The model under review builds one solid part; all positions refer to its coordinate system, in mm. A direction names the side the tool comes from. Coordinates: 2 decimals unless noted, no trailing zeros. Loops run counter-clockwise (first coordinate to the right, second up) from the corner with the lowest first, then second, coordinate; pieces in that order, holes last. Notation, with made-up numbers: (22, -16) - (78, -16) arc R19 cw to (78, 3) - close; hole circle Ø3 at (34.5, 59). An arc over 180 degrees is marked (long way). Answer in a Markdown table with one row per item. Add a question column.
(1) For line 1 along X through (y, z) = (-0.5, 1.45); line 2 along Z through (x, y) = (-2, -1.5); line 3 along X through (y, z) = (3.75, 2.3), list the stretches that pass through material, from the lowest coordinate up.
(2) Machinability: for faces 4 (the flat face through (1.3, -0.1, 1.8)), 5 (the flat face through (-0.21, -5, 0.48)), which of the approach directions +Z, -Z, +X, -X, +Y, -Y give a long, thin tool a straight path to every point of the face, cutting with its end or side? Answer none if there is none.
(3) Mouldability with a two-part tool opening along X and no side actions: class faces 1 (the flat face through (0, 0, 0)), 2 (the flat face through (-15, 0, 1)), 3 (the flat face through (-1.2, -0.1, 1.7)) as +X half, -X half, draft (parallel to the pull), parting line (faces both ways), or undercut.
(4) We need section A-A on z = 1.3. Write out the cut boundary in (x, y).
(5) We need section B-B on y = -3.5. Write out the cut boundary in (x, z).
(6) We need section C-C on x = -0.5. Write out the cut boundary in (y, z).
from build123d import *

# Parameters (mm, degrees)
SKETCH_W     = 30
SKETCH_H     = 10
PAD_DEPTH    = 3
POCKET_DEPTH = 10.001


with BuildPart() as part:
    # Sketch → Pad (new body)
    with BuildSketch(Plane.XY):
        Rectangle(SKETCH_W, SKETCH_H)
    extrude(amount=PAD_DEPTH)

    # Sketch001 (on Face2 of Pad) → Pocket (cut, through all)
    with BuildSketch(Plane.XZ.offset(5)):
        Polygon((0, 0.5), (-2.5, 3), (2.5, 3), align=None)
    extrude(amount=-POCKET_DEPTH, mode=Mode.SUBTRACT)


solid = part.part
Outcome:
| question | item | result |
|---|---|---|
| 1 | line 1 | -15 to -0.95, 0.95 to 15 |
| 1 | line 2 | 0 to 2.5 |
| 1 | line 3 | -15 to -1.8, 1.8 to 15 |
| 2 | face 4 | +Z, +Y, -Y |
| 2 | face 5 | +Z, -Z, +X, -X, -Y |
| 3 | face 1 | draft |
| 3 | face 2 | -X half |
| 3 | face 3 | undercut |
| 4 | outline | (-15, -5) - (-0.8, -5) - (-0.8, 5) - (-15, 5) - close; (0.8, -5) - (15, -5) - (15, 5) - (0.8, 5) - close |
| 5 | outline | (-15, 0) - (15, 0) - (15, 3) - (2.5, 3) - (0, 0.5) - (-2.5, 3) - (-15, 3) - close |
| 6 | outline | (-5, 0) - (5, 0) - (5, 1) - (-5, 1) - close |
